Part model, mm, in its own coordinate system. A direction names the side the tool comes from. Round coordinates to 2 decimals unless told otherwise and drop trailing zeros. Write each loop counter-clockwise with the first axis right and the second up, starting at its lowest first coordinate (ties: lowest second). Pieces come first, ordered by that corner, then holes. Notation, with made-up numbers: (-36.75, -35) -> (3.25, -35) arc R24 cw to (3.25, -5) -> close; hole circle Ø1 at (63.5, -26.5). An arc over 180 degrees is marked (long way). Return JSON: item names as keys, results as strings. Group by question number.
(1) Tool access for faces 1 (the flat face through (5, -5, 2)), 2 (the flat face through (0, 0, 0)): list every direction of +Z, -Z, +X, -X, +Y, -Y with a clear straight run to the whole face (end or side of a thin tool).
(2) Saw through at A-A (y = 0). List the corners of the cut face in (x, z).
(3) Saw through at D-D (z = 0.45). List the corners of the cut face in (x, y).
(4) Drop flat-ended pins along their axis: pin 1 Ø1 at (x, z) = (2.5, 1.5) entering from +Y; pin 2 Ø2 at (y, z) = (3.5, 1.5) entering from +X (3 decimals). Give the stop position or say it passes through.
(5) Saw through at C-C (z = 5.05). List the corners of the cut face in (x, y), plus the area to 3 significant figures.
(6) Drill centre lines: L1, parallel to Z at x = -4.5, y = -9.25; L2, parallel to X at y = -0.25, z = 5.1; L3, parallel to Z at x = -0.25, y = 5.5. Where is each one in solid material? Low to high. Write a range as from..to.
from build123d import *

# Parameters (mm, degrees)
F0_R     = 12.5
F1_DEPTH = 2
F2_R     = 1
F3_R     = 6
F4_DEPTH = 0.5
F5_R     = 4
F6_DEPTH = 3


with BuildPart() as f1:
    # F0 (on Top) → F1 (new body)
    with BuildSketch(Plane.XY):
        Circle(F0_R)
    extrude(amount=F1_DEPTH)

    # F2
    f2_edges = [f1.edges().sort_by_distance(p)[0] for p in [
        (-12.5, 0, 2),
    ]]
    fillet(f2_edges, radius=F2_R)

    # F3 (on face) → F4 (join)
    with BuildSketch(Plane.XY.offset(2)):
        Circle(F3_R)
    extrude(amount=F4_DEPTH)

    # F5 (on face) → F6 (join)
    with BuildSketch(Plane.XY.offset(2.5)):
        Circle(F5_R)
    extrude(amount=F6_DEPTH)


solid = f1.part
Computed values:
{
 "1": {"face 1": "+Z", "face 2": "-Z, +X, -X, +Y, -Y"},
 "2": {"outline": "(-12.5, 0) -> (12.5, 0) -> (12.5, 1) arc R1 ccw to (11.5, 2) -> (6, 2) -> (6, 2.5) -> (4, 2.5) -> (4, 5.5) -> (-4, 5.5) -> (-4, 2.5) -> (-6, 2.5) -> (-6, 2) -> (-11.5, 2) arc R1 ccw to (-12.5, 1) -> close"},
 "3": {"outline": "circle Ø25 at (0, 0)"},
 "4": {"pin 1": "y = 12.3", "pin 2": "x = 12.225"},
 "5": {"outline": "circle Ø8 at (0, 0)", "area": "50.3 mm2"},
 "6": {"L1": "0..2", "L2": "-3.99..3.99", "L3": "0..2.5"}
}
